```python
from build123d import *

# Parameters (mm, degrees)
MAIN_PLATE_DEPTH                = 5.3
F_4_0MM_CLEARANCE_DOWEL_HOLE1_D = 4
F_4_0MM_CLEARANCE_DOWEL_HOLE2_D = 4
F_3_0MM_PRESS_DOWEL_HOLE1_D     = 2.54
CUT_EXTRUDE1_DEPTH              = 6.3


with BuildPart() as part:
    # Sketch1 → Main Plate (new body)
    with BuildSketch(Plane(origin=(0, 0, 0), x_dir=(1, 0, 0), z_dir=(0, 1, 0))):
        Polygon((-146.05, -95.25), (146.05, -95.25), (146.05, -12.7), (146.05, 12.7), (146.05, 95.25), (-146.05, 95.25), (-146.05, 12.7), (-146.05, -12.7), align=None)
    extrude(amount=MAIN_PLATE_DEPTH)

    # Ø4.0mm Clearance Dowel Hole1 (through all)
    with Locations(Plane(origin=(0, 5.3, 0), x_dir=(1, 0, 0), z_dir=(0, 1, 0))):
        with Locations((109.17919222, -46.780829645), (72.308384441, -46.780829645), (36.5125, -47.202914823), (109.17919222, 0), (72.308384441, 0), (36.15419222, 0), (109.17919222, 47.625), (72.308384441, 47.625), (36.15419222, 47.625), (0, 47.625), (-36.5125, 47.625), (-73.025, 47.625), (-109.5375, 47.625), (-109.5375, 0), (-73.025, 0), (-36.5125, 0), (0, 0), (0, -47.625), (-36.5125, -47.625), (-73.025, -47.625), (-109.5375, -47.625)):
            Hole(F_4_0MM_CLEARANCE_DOWEL_HOLE1_D / 2)

    # Ø4.0mm Clearance Dowel Hole2 (through all)
    with Locations(Plane(origin=(0, 5.3, 0), x_dir=(1, 0, 0), z_dir=(0, 1, 0))):
        with Locations((5, -85.25), (-5, -85.25), (-136.05, -5), (-136.05, 5), (5, 85.25), (-5, 85.25), (134.05, -5), (134.05, 5)):
            Hole(F_4_0MM_CLEARANCE_DOWEL_HOLE2_D / 2)

    # Ø3.0mm Press Dowel Hole1 (through all)
    with Locations(Plane(origin=(0, 5.3, 0), x_dir=(1, 0, 0), z_dir=(0, 1, 0))):
        with Locations((-19.96, 7.07), (-19.96, -7.07), (19.96, 7.07), (19.96, -7.07)):
            Hole(F_3_0MM_PRESS_DOWEL_HOLE1_D / 2)

    # Sketch12 → Cut-Extrude1 (cut, through all)
    with BuildSketch(Plane(origin=(0, 5.3, 0), x_dir=(1, 0, 0), z_dir=(0, 1, 0))):
        Polygon((146.05, -63.5), (114.3, -95.25), (146.05, -95.25), align=None)
        Polygon((-114.3, -95.25), (-146.05, -63.5), (-146.05, -95.25), align=None)
        Polygon((-146.05, 95.25), (-146.05, 63.5), (-114.3, 95.25), align=None)
        Polygon((146.05, 95.25), (114.3, 95.25), (146.05, 63.5), align=None)
    extrude(amount=-CUT_EXTRUDE1_DEPTH, mode=Mode.SUBTRACT)


solid = part.part
```
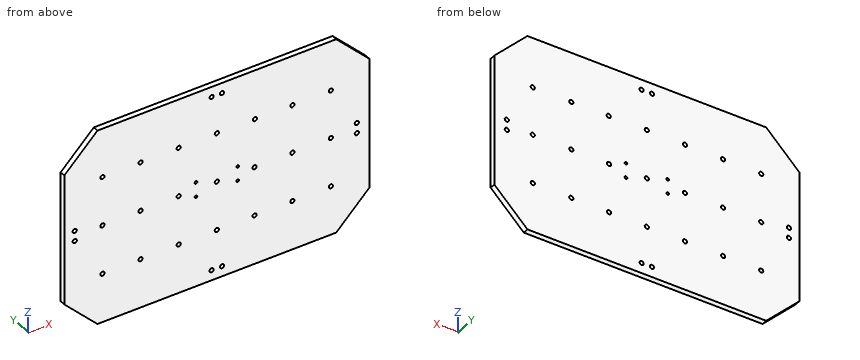
Geometry: final body of the model. Coordinates: model frame, mm. Give positions to 0.01 mm unless a question says otherwise; leave off trailing zeros. Order: outer loops, then holes, each group sorted by start corner. A loop starts at its lowest first (then second) coordinate and runs counter-clockwise, first axis right, second up. Notation, with made-up numbers: (82, 76) -> (105, 76) arc R19 ccw to (105, 95) -> close; hole circle Ø4 at (81, -36.5). An arc over 180 degrees is marked (long way). Write each question's results on one line, items separated by ' | '. Start each with the question number.
1) Section A-A (z = 72.5). Return loops of the section in (x, y), then the cut area to 3 significant figures.
2) Line query: line 1 (Z direction, x = 19.96, y = 2.95); line 2 (Z direction, x = -5, y = 1.25); line 3 (X direction, y = 0.75, z = 86). Output: solid intervals per line, ascending. Write a range as from..to.
3) First-contact query: pin 1 (2.5 mm diameter, centred on x = -109.54, z = 47.62, fed in from -Y). Flat tip, straight axial feed; report the tip coordinate or a pass-through.
4) Section B-B (y = 2.75). Count the separate pieces of the cut face and the enclosed holes in it, then the cut area to 3 significant figures.
Calculated:
1) outline: (-137.05, 0) -> (137.05, 0) -> (137.05, 5.3) -> (-137.05, 5.3) -> close | area: 1,450 mm2
2) line 1: -95.25..-8.34, -5.8..5.8, 8.34..95.25 | line 2: -95.25..-87.25, -83.25..83.25, 87.25..95.25 | line 3: -123.55..-6.85, -3.15..3.15, 6.85..123.55
3) pin 1: through
4) separate pieces: 1 | enclosed holes: 33 | area: 53,200 mm2
